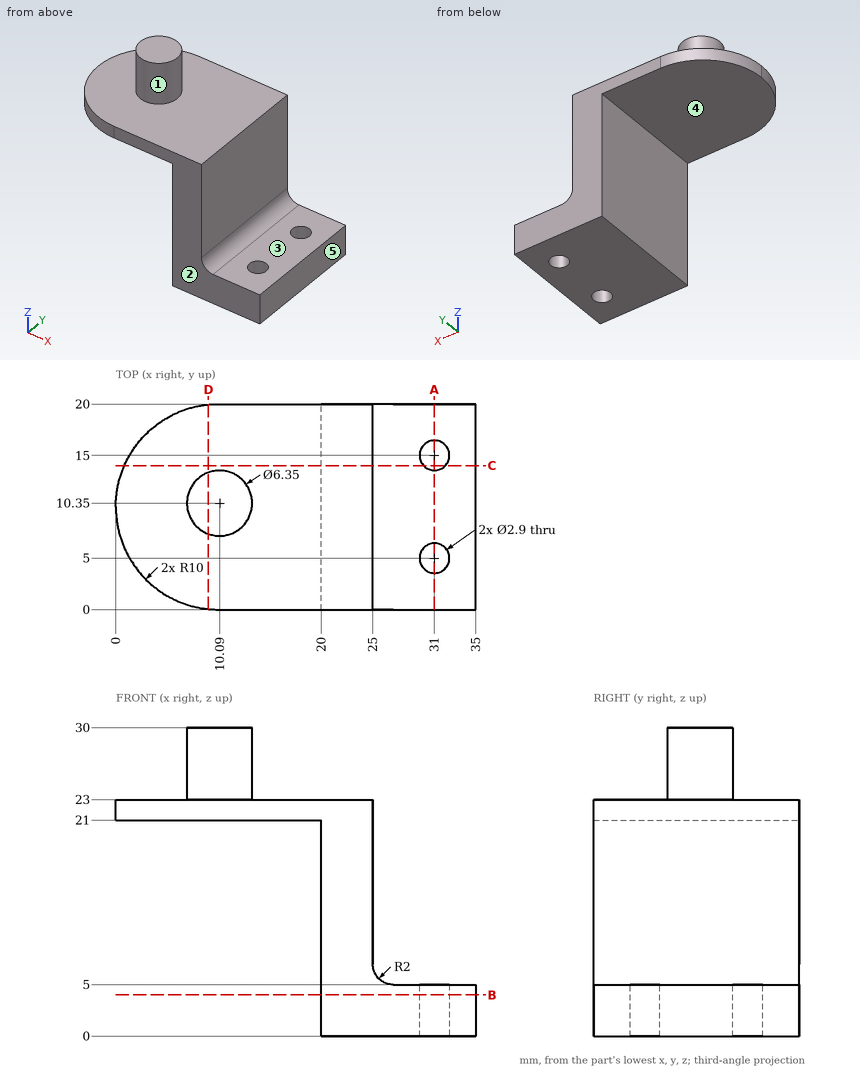
Print and shaded views of the part. All mm, measured from the part's lowest x, y and z. A direction names the side the tool comes from. Round coordinates to 2 decimals unless told otherwise and drop trailing zeros. Write each loop counter-clockwise with the first axis right and the second up, starting at its lowest first coordinate (ties: lowest second). Pieces come first, ordered by that corner, then holes. Notation, with made-up numbers: (-18.5, 14) -> (12.5, 14) arc R28 ccw to (12.5, 43) -> close; hole circle Ø2 at (-21, 21.5). An arc over 180 degrees is marked (long way). Return JSON: item names as keys, results as strings. Group by question number.
Q1. Probe L1, parallel to Y at x = 31, z = 2; L2, parallel to Z at x = 2.5, y = 8.25; L3, parallel to Z at x = 11.5, y = 8.75. List the from-to ranges inside material, lowest first. Write a range as [from, to].
Q2. Saw through at C-C on y = 14. Write the cut outline in (x, z) (3 decimals), plus the area to 3 significant figures.
Q3. Pin check, flat tips, straight feed: pin 1 (5 mm diameter, centred on x = 4.5, y = 15.5, fed in from -Z); pin 2 (6.5 mm diameter, centred on x = 32.5, y = 9, fed in from +Z); pin 3 (8 mm diameter, centred on y = 16, z = 16.5, fed in from -X); pin 4 (1.7 mm diameter, centred on x = 31, y = 15, fed in from -Z). Stop position of each tip, or through.
Q4. Saw through at D-D on x = 9. Write the cut outline in (y, z).
Q5. Saw through at A-A on x = 31. Write the cut outline in (y, z).
Q6. Saw through at B-B on z = 4. Write the cut outline in (x, y), plus the area to 3 significant figures.
Q7. Which spindle directions (+Z, -Z, +X, -X, +Y, -Y) get a long thin tool onto all of the face, cutting with end or side? Do the marked faces 1, 2, 3, 4 and 5. Say none if no direction does.
Answer:
{
 "1": {"L1": "[0, 3.55], [6.45, 13.55], [16.45, 20]", "L2": "[21, 23]", "L3": "[21, 30]"},
 "2": {"outline": "(0.835, 21) -> (20, 21) -> (20, 0) -> (29.95, 0) -> (29.95, 5) -> (27, 5) arc R2 cw to (25, 7) -> (25, 23) -> (0.835, 23) -> close; (32.05, 0) -> (35, 0) -> (35, 5) -> (32.05, 5) -> close", "area": "194 mm2"},
 "3": {"pin 1": "z = 21", "pin 2": "z = 5", "pin 3": "x = 20", "pin 4": "through"},
 "4": {"outline": "(0.05, 21) -> (19.95, 21) -> (19.95, 23) -> (13.33, 23) -> (13.33, 30) -> (7.37, 30) -> (7.37, 23) -> (0.05, 23) -> close"},
 "5": {"outline": "(0, 0) -> (3.55, 0) -> (3.55, 5) -> (0, 5) -> close; (6.45, 0) -> (13.55, 0) -> (13.55, 5) -> (6.45, 5) -> close; (16.45, 0) -> (20, 0) -> (20, 5) -> (16.45, 5) -> close"},
 "6": {"outline": "(20, 0) -> (35, 0) -> (35, 20) -> (20, 20) -> close; hole circle Ø2.9 at (31, 5); hole circle Ø2.9 at (31, 15)", "area": "287 mm2"},
 "7": {"face 1": "+Z", "face 2": "+Z, -Z, +X, -X, -Y", "face 3": "+Z, +X, +Y, -Y", "face 4": "-Z, -X, +Y, -Y", "face 5": "+Z, -Z, +X, +Y, -Y"}
}
